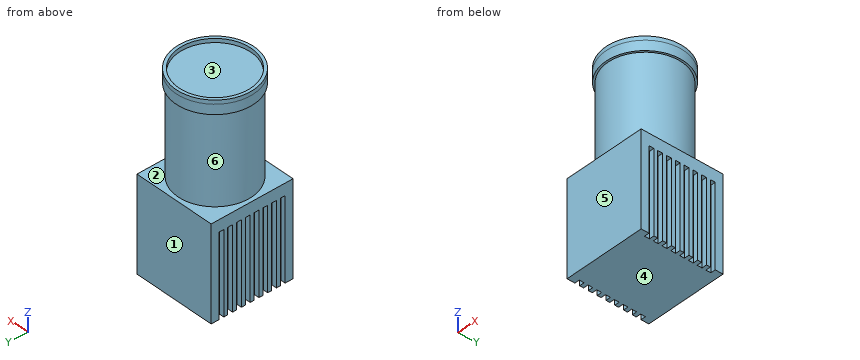
```python
from build123d import *

# Parameters (mm, degrees)
SKETCH2_W           = 42
SKETCH2_H           = 42
BOSS_EXTRUDE1_DEPTH = 48
SKETCH3_R           = 19
BOSS_EXTRUDE2_DEPTH = 50
SKETCH4_R           = 20
SKETCH4_R_2         = 18.5
BOSS_EXTRUDE3_DEPTH = 5
SKETCH5_R           = 20
SKETCH5_R_2         = 18.5
BOSS_EXTRUDE4_DEPTH = 2
SKETCH6_W           = 2.5
SKETCH6_H           = 2.5
CUT_EXTRUDE1_DEPTH  = 42


with BuildPart() as part:
    # Sketch2 → Boss-Extrude1 (new body)
    with BuildSketch(Plane.XY):
        with Locations((21, 21)):
            Rectangle(SKETCH2_W, SKETCH2_H)
    extrude(amount=BOSS_EXTRUDE1_DEPTH)

    # Sketch3 → Boss-Extrude2 (add)
    with BuildSketch(Plane.XY.offset(48)):
        with Locations((21, 21)):
            Circle(SKETCH3_R)
    extrude(amount=BOSS_EXTRUDE2_DEPTH)



with BuildPart() as body_2:
    # Sketch4 → Boss-Extrude3 (new body)
    with BuildSketch(Plane.XY.offset(98)):
        with Locations((21, 21)):
            Circle(SKETCH4_R)
        with Locations((21, 21)):
            Circle(SKETCH4_R_2, mode=Mode.SUBTRACT)
    extrude(amount=-BOSS_EXTRUDE3_DEPTH)


with BuildPart() as part_1:
    add(part.part)

    add(body_2.part)  # Boss-Extrude4 merges body 2
    # Sketch5 → Boss-Extrude4 (add)
    with BuildSketch(Plane.XY.offset(98)):
        with Locations((21, 21)):
            Circle(SKETCH5_R)
        with Locations((21, 21)):
            Circle(SKETCH5_R_2, mode=Mode.SUBTRACT)
    extrude(amount=BOSS_EXTRUDE4_DEPTH)

    # Sketch6 → Cut-Extrude1 (cut)
    with BuildSketch(Plane(origin=(0, 0, 0), x_dir=(-1, 0, 0), z_dir=(0, 0, -1))):
        with Locations((-40.75, 36.75)):
            Rectangle(SKETCH6_W, SKETCH6_H)
        with Locations((-40.75, 5.25)):
            Rectangle(SKETCH6_W, SKETCH6_H)
        with Locations((-40.75, 32.25)):
            Rectangle(SKETCH6_W, SKETCH6_H)
        with Locations((-40.75, 23.25)):
            Rectangle(SKETCH6_W, SKETCH6_H)
        with Locations((-40.75, 18.75)):
            Rectangle(SKETCH6_W, SKETCH6_H)
        with Locations((-40.75, 14.25)):
            Rectangle(SKETCH6_W, SKETCH6_H)
        with Locations((-40.75, 9.75)):
            Rectangle(SKETCH6_W, SKETCH6_H)
        with Locations((-40.75, 27.75)):
            Rectangle(SKETCH6_W, SKETCH6_H)
        with Locations((-1.25, 5.25)):
            Rectangle(SKETCH6_W, SKETCH6_H)
        with Locations((-1.25, 27.75)):
            Rectangle(SKETCH6_W, SKETCH6_H)
        with Locations((-1.25, 9.75)):
            Rectangle(SKETCH6_W, SKETCH6_H)
        with Locations((-1.25, 14.25)):
            Rectangle(SKETCH6_W, SKETCH6_H)
        with Locations((-1.25, 18.75)):
            Rectangle(SKETCH6_W, SKETCH6_H)
        with Locations((-1.25, 23.25)):
            Rectangle(SKETCH6_W, SKETCH6_H)
        with Locations((-1.25, 32.25)):
            Rectangle(SKETCH6_W, SKETCH6_H)
        with Locations((-1.25, 36.75)):
            Rectangle(SKETCH6_W, SKETCH6_H)
    extrude(amount=-CUT_EXTRUDE1_DEPTH, mode=Mode.SUBTRACT)


solid = part_1.part
```
Can you work these out from the model? Positions are in its coordinate system, mm. Face numbers are marked on the shaded views. A direction names the side the tool comes from. Coordinates: 2 decimals unless noted, no trailing zeros. Write each loop counter-clockwise with the first axis right and the second up, starting at its lowest first coordinate (ties: lowest second). Pieces come first, ordered by that corner, then holes. Notation, with made-up numbers: M 85.25,-30 L 123.25,-30 A22 ccw 123.25,-5 Z; hole C 14,34.5 d1. An arc over 180 degrees is marked long. Write item = value, one per line. Start each with the question number.
Q1. On a 3-axis mill with a long thin cutter (end or side, diameter ignored), from which of +Z, -Z, +X, -X, +Y, -Y can I reach the whole of each face in a straight line? I mean the marked faces 1 and 2. Say none if no direction works.
Q2. If I drill on L1, parallel to Y at x = 21, z = 99.1; L2, parallel to Z at x = 28, y = 28; L3, parallel to Z at x = 3.5, y = 29.5, over which ranges is the centre line in solid material (lowest first)? Write a range as [from, to].
Q3. Thinking about a two-plate mould opening in Z: for the marked faces 3, 4, 5 and 6, which applies, released by +Z, released by -Z, zero draft, split by the parting line, or undercut?
Q4. If we section it at A-A, the plane y = 21: Write out the boundary of the cut face in (x, z), then the cut area to 3 significant figures.
Q5. I'm going to push flat-ended pins straight in: pin 1 (4 mm diameter, centred on x = 12, y = 16.5, fed in from -Z); pin 2 (1.2 mm diameter, centred on x = 1.5, y = 18.5, fed in from -Z); pin 3 (6 mm diameter, centred on x = 17.5, z = 67, fed in from +Y); pin 4 (11 mm diameter, centred on x = 15.5, y = 25, fed in from +Z). Where does each tip first touch, or does it pass through?
Check sheet entries:
q1.face_1 = +Z, -Z, +X, -X, +Y
q1.face_2 = none
q2.L1 = [1, 2.5], [39.5, 41]
q2.L2 = [0, 98]
q2.L3 = [0, 48], [93, 100]
q3.face_3 = released by +Z
q3.face_4 = released by -Z
q3.face_5 = zero draft
q3.face_6 = undercut
q4.outline = M 0,0 L 42,0 L 42,48 L 40,48 L 40,93 L 41,93 L 41,100 L 39.5,100 L 39.5,98 L 2.5,98 L 2.5,100 L 1,100 L 1,93 L 2,93 L 2,48 L 0,48 Z
q4.area = 3,930 mm²
q5.pin_1 = 0
q5.pin_2 = 42
q5.pin_3 = 39.99
q5.pin_4 = 98
